```python
from build123d import *

# Parameters (mm, degrees)
BOSS_EXTRUDE1_DEPTH = 3.175
FILLET1_R           = 1
FILLET2_R           = 1
CHAMFER1_SIZE       = 1


with BuildPart() as part:
    # Sketch1 → Boss-Extrude1 (new body)
    with BuildSketch(Plane.XY):
        with BuildLine():
            Line((0, 0), (-45.974, -79.629303827))
            ThreePointArc((-45.974, -79.629303827), (-43.649738686, -88.303565141), (-34.975477372, -85.979303827))
            Line((-34.975477372, -85.979303827), (0, -25.4))
            Line((0, -25.4), (34.975477372, -85.979303827))
            ThreePointArc((34.975477372, -85.979303827), (43.649738686, -88.303565141), (45.974, -79.629303827))
            Line((45.974, -79.629303827), (0, 0))
        make_face()
        with BuildLine():
            Line((-1.139014765, -8.322831444), (-9.950369343, -23.584545256))
            ThreePointArc((-9.950369343, -23.584545256), (-8.788238686, -27.921675913), (-4.451108029, -26.759545256))
            Line((-4.451108029, -26.759545256), (-2.749630657, -23.8125))
            Line((-2.749630657, -23.8125), (-1.374815329, -21.43125))
            Line((-1.374815329, -21.43125), (-1.139014765, -8.322831444))
        make_face(mode=Mode.SUBTRACT)
        with BuildLine():
            Line((-38.1, -72.341135768), (-43.224369343, -81.216803827))
            ThreePointArc((-43.224369343, -81.216803827), (-42.062238686, -85.553934484), (-37.725108029, -84.391803827))
            Line((-37.725108029, -84.391803827), (-32.600738686, -75.516135768))
            ThreePointArc((-32.600738686, -75.516135768), (-35.775738686, -74.665397082), (-38.1, -72.341135768))
        make_face(mode=Mode.SUBTRACT)
        with BuildLine():
            Line((-19.900738686, -53.519090512), (-29.851108029, -70.753635768))
            ThreePointArc((-29.851108029, -70.753635768), (-34.188238686, -71.915766425), (-35.350369343, -67.578635768))
            Line((-35.350369343, -67.578635768), (-25.4, -50.344090512))
            ThreePointArc((-25.4, -50.344090512), (-23.075738686, -52.668351826), (-19.900738686, -53.519090512))
        make_face(mode=Mode.SUBTRACT)
        with BuildLine():
            Line((-7.200738686, -31.522045256), (-17.151108029, -48.756590512))
            ThreePointArc((-17.151108029, -48.756590512), (-21.488238686, -49.918721169), (-22.650369343, -45.581590512))
            Line((-22.650369343, -45.581590512), (-12.7, -28.347045256))
            ThreePointArc((-12.7, -28.347045256), (-10.375738686, -30.67130657), (-7.200738686, -31.522045256))
        make_face(mode=Mode.SUBTRACT)
        with BuildLine():
            Line((2.749630657, -23.8125), (1.374815329, -21.43125))
            Line((1.374815329, -21.43125), (1.139014765, -8.322831444))
            Line((1.139014765, -8.322831444), (9.950369343, -23.584545256))
            ThreePointArc((9.950369343, -23.584545256), (8.788238686, -27.921675913), (4.451108029, -26.759545256))
            Line((4.451108029, -26.759545256), (2.749630657, -23.8125))
        make_face(mode=Mode.SUBTRACT)
        with BuildLine():
            Line((12.7, -28.347045256), (22.650369343, -45.581590512))
            ThreePointArc((22.650369343, -45.581590512), (21.488238686, -49.918721169), (17.151108029, -48.756590512))
            Line((17.151108029, -48.756590512), (7.200738686, -31.522045256))
            ThreePointArc((7.200738686, -31.522045256), (10.375738686, -30.67130657), (12.7, -28.347045256))
        make_face(mode=Mode.SUBTRACT)
        with BuildLine():
            Line((25.4, -50.344090512), (35.350369343, -67.578635768))
            ThreePointArc((35.350369343, -67.578635768), (34.188238686, -71.915766425), (29.851108029, -70.753635768))
            Line((29.851108029, -70.753635768), (19.900738686, -53.519090512))
            ThreePointArc((19.900738686, -53.519090512), (23.075738686, -52.668351826), (25.4, -50.344090512))
        make_face(mode=Mode.SUBTRACT)
        with BuildLine():
            Line((32.600738686, -75.516135768), (37.725108029, -84.391803827))
            Line((37.725108029, -84.391803827), (41.041728895, -77.436359677))
            Line((41.041728895, -77.436359677), (38.1, -72.341135768))
            ThreePointArc((38.1, -72.341135768), (35.775738686, -74.665397082), (32.600738686, -75.516135768))
        make_face(mode=Mode.SUBTRACT)
        with BuildLine():
            Line((39.510088039, -85.709715542), (42.266670891, -79.871944556))
            Line((42.266670891, -79.871944556), (42.348213443, -79.699257294))
            Line((42.348213443, -79.699257294), (43.224369343, -81.216803827))
            ThreePointArc((43.224369343, -81.216803827), (42.931408354, -84.815621589), (39.461225977, -85.813193487))
            Line((39.461225977, -85.813193487), (39.510088039, -85.709715542))
        make_face(mode=Mode.SUBTRACT)
    extrude(amount=BOSS_EXTRUDE1_DEPTH)

    # Fillet1
    fillet1_edges = [part.edges().sort_by_distance(p)[0] for p in [
        (0, 0, 1.5875),
        (-1.139014765, -8.322831444, 1.5875),
        (1.139014765, -8.322831444, 1.5875),
    ]]
    fillet(fillet1_edges, radius=FILLET1_R)

    # Fillet2
    fillet2_edges = [part.edges().sort_by_distance(p)[0] for p in [
        (0, -25.4, 1.5875),
    ]]
    fillet(fillet2_edges, radius=FILLET2_R)

    # Chamfer1
    chamfer1_edges = [part.edges().sort_by_distance(p)[0] for p in [
        (-43.649738686, -88.303565141, 3.175),
        (-17.920751388, -56.439651914, 3.175),
        (-23.420012702, -40.564651914, 3.175),
        (0, -1, 3.175),
        (17.920751388, -56.439651914, 3.175),
        (0, -26.4, 3.175),
        (43.649738686, -88.303565141, 3.175),
        (23.420012702, -40.564651914, 3.175),
    ]]
    chamfer(chamfer1_edges, length=CHAMFER1_SIZE - 0.0001)  # a hair under: the kernel refuses the full size


solid = part.part
```
Here's how the part is built. I have some questions about the finished solid (model axes, mm). A direction names the side the tool comes from. Coordinates: 2 decimals unless noted, no trailing zeros. Loops run counter-clockwise (first coordinate to the right, second up) from the corner with the lowest first, then second, coordinate; pieces in that order, holes last. Notation, with made-up numbers: (48, -20) -> (82, -20) arc R30 cw to (82, 11) -> close; hole circle Ø11 at (50, 66). An arc over 180 degrees is marked (long way). Return JSON: item names as keys, results as strings.
1) If we section it at A-A, the plane y = -19: Write out the boundary of the cut face in (x, z) (3 decimals), then the cut area to 3 significant figures.
Results below:
{"outline": "(-10.97, 0) -> (-7.303, 0) -> (-7.303, 3.175) -> (-9.815, 3.175) -> (-10.97, 2.175) -> close; (-1.331, 0) -> (1.331, 0) -> (1.331, 3.175) -> (-1.331, 3.175) -> close; (7.303, 0) -> (10.97, 0) -> (10.97, 2.175) -> (9.815, 3.175) -> (7.303, 3.175) -> close", "area": "30.6 mm²"}
2) If we section it at C-C, the plane y = -38: Write out the boundary of the cut face in (x, z) (3 decimals), then the cut area to 3 significant figures.
Results below:
{"outline": "(-21.939, 0) -> (-18.273, 0) -> (-18.273, 3.175) -> (-20.785, 3.175) -> (-21.939, 2.175) -> close; (-10.941, 0) -> (-7.275, 0) -> (-7.275, 2.175) -> (-8.429, 3.175) -> (-10.941, 3.175) -> close; (7.275, 0) -> (10.941, 0) -> (10.941, 3.175) -> (8.429, 3.175) -> (7.275, 2.175) -> close; (18.273, 0) -> (21.939, 0) -> (21.939, 2.175) -> (20.785, 3.175) -> (18.273, 3.175) -> close", "area": "44.3 mm²"}
3) Will these pins go through, and if not, where does the flat tip stop? pin 1 (4 mm diameter, centred on x = -15.5, y = -45, fed in from +Z) (3 decimals); pin 2 (1.5 mm diameter, centred on x = -22, z = 1, fed in from -Y); pin 3 (5 mm diameter, centred on x = 3, y = -37.5, fed in from +Z).
Results below:
{"pin 1": "z = 3.175", "pin 2": "y = -64.8", "pin 3": "through"}
4) If we section it at B-B, the plane x = -6: Write out the boundary of the cut face in (y, z) (1 decimal).
Results below:
{"outline": "(-35.8, 0) -> (-28.1, 0) -> (-28.1, 3.2) -> (-33.8, 3.2) -> (-35.8, 2.2) -> close; (-16.7, 0) -> (-10.4, 0) -> (-10.4, 2.2) -> (-12.4, 3.2) -> (-16.7, 3.2) -> close"}
5) Thinking about a two-plate mould opening in X: for faces 3 (the face through (-40.63, -76.72, 1.57)), 4 (the face through (-23.104, -40.018, 1.072)), which applies, +X half, -X half, draft (parallel to the pull), parting line (faces both ways), or undercut?
Results below:
{"face 3": "undercut", "face 4": "-X half"}
6) If we section it at D-D, the plane z = 0.6: Count the separate pieces of the cut face and the enclosed holes in it, then the cut area to 3 significant figures.
Results below:
{"separate pieces": "1", "enclosed holes": "9", "area": "1,310 mm²"}
7) For faces 1 (the face through (30.306, -58.841, 1.565)), 2 (the face through (-18.16, -56.853, 1.072)), which set-ups out of +Z, -Z, +X, -X, +Y, -Y let a thin tool reach every point of the face, with its end or its side?
Results below:
{"face 1": "+Z, -Z", "face 2": "+Z, -Z, -Y"}
8) I need wall thicknesses on line 1 (Y direction, x = -20, z = 0.4); line 2 (X direction, y = -81.5, z = 1.2); line 3 (Y direction, x = 41, z = 2). Which ranges of each line are inside material? Lowest first, please. Write a range as from..to.
Results below:
{"line 1": "-60.04..-53.69, -53.52..-50.34, -40.99..-34.64", "line 2": "-46.69..-43.37, -36.06..-32.39, 32.39..36.06, 39.1..41.5, 43.37..46.69", "line 3": "-89.13..-85.94, -82.55..-77.52, -77.36..-71.01"}
